from build123d import *

# Parameters (mm, degrees)
SKETCH1_W                 = 270.7
SKETCH1_H                 = 127
SKETCH1_R                 = 1.6
WALL_DEPTH                = 6.35
SKETCH5_R                 = 3.96875
RODSUPPORTCUTOUT_DEPTH    = 3.175
SUPPORTPATTERN_COUNT      = 7
SUPPORTPATTERN_PITCH      = 36.65
SUPPORTPATTERN_COUNT_DIR2 = 5
SUPPORTPATTERN_PITCH_DIR2 = 19.05


with BuildPart() as part:
    # Sketch1 → Wall (new body)
    with BuildSketch(Plane.XY):
        with Locations((135.35, 63.5)):
            Rectangle(SKETCH1_W, SKETCH1_H)
        with Locations((12.35, 105)):
            Circle(SKETCH1_R, mode=Mode.SUBTRACT)
        with Locations(Location((258.35, 105, 0), (0, 0, 180))):
            Circle(SKETCH1_R, mode=Mode.SUBTRACT)
        with Locations((258.35, 22)):
            Circle(SKETCH1_R, mode=Mode.SUBTRACT)
        with Locations(Location((12.35, 22, 0), (0, 0, 180))):
            Circle(SKETCH1_R, mode=Mode.SUBTRACT)
    extrude(amount=WALL_DEPTH)

    # Sketch5 → RodSupportCutout (cut)
    with BuildSketch(Plane.XY.offset(6.35)):
        with Locations(Location((25.4, 101.6, 0), (0, 0, 180))):
            Circle(SKETCH5_R)
    rodsupportcutout = extrude(amount=-RODSUPPORTCUTOUT_DEPTH, mode=Mode.SUBTRACT)

    # SupportPattern: RodSupportCutout 7 × 5
    with Locations(*[(i * SUPPORTPATTERN_PITCH, -j * SUPPORTPATTERN_PITCH_DIR2, 0) for i in range(SUPPORTPATTERN_COUNT) for j in range(SUPPORTPATTERN_COUNT_DIR2) if (i, j) != (0, 0)]):
        add(rodsupportcutout, mode=Mode.SUBTRACT)


solid = part.part
Read the model definition and answer for the solid it produces. Units are mm, in the model's axes. A direction names the side the tool comes from. Round coordinates to 2 decimals unless told otherwise and drop trailing zeros. Order: outer loops, then holes, each group sorted by start corner. A loop starts at its lowest first (then second) coordinate and runs counter-clockwise, first axis right, second up. Notation, with made-up numbers: (69, 32.25) - (93, 32.25) arc R19 ccw to (93, 55.25) - close; hole circle Ø7 at (40, -23). An arc over 180 degrees is marked (long way). Use one line per item in the form item = value. Start each with the question number.
(1) Determine the mould class of faces 3 (the face through (133, 0, 3)), 4 (the face through (101.625, 60.818, 4.785)), 5 (the face through (270.7, 63, 3)) for opening direction X: +X half, -X half, draft (parallel to the pull), parting line (faces both ways), or undercut.
(2) The part is cut by section C-C (x = 209.5). Give the vertices of the cut face in (y, z) (3 decimals), then the cut area to 3 significant figures.
(3) The part is cut by section A-A (x = 98.7). Give the vertices of the cut face in (y, z) (3 decimals).
(4) For faces 1 (the face through (133, 127, 3)), 2 (the face through (209, 44, 3.175)), determine the directions among +Z, -Z, +X, -X, +Y, -Y from which every point of the face is accessible in a straight line to the end or side of a thin tool.
(5) Flat-ended cylindrical pins translate along their axes: pin 1 Ø6.5 at (x, y) = (246, 103) entering from +Z; pin 2 Ø6.5 at (x, y) = (172, 25.4) entering from +Z (3 decimals). Find the tip coordinate at first contact, or state that the pin passes through.
(6) Find the intervals of material crossed by line 1 along Y through (x, z) = (136, 5.25); line 2 along Y through (x, z) = (208.65, 4.85); line 3 along X through (y, z) = (105, 2), in increasing order. Write a range as from..to.
Checked values:
q1.face_3 = draft
q1.face_4 = undercut
q1.face_5 = +X half
q2.outline = (0, 0) - (127, 0) - (127, 6.35) - (105.477, 6.35) - (105.477, 3.175) - (97.723, 3.175) - (97.723, 6.35) - (86.427, 6.35) - (86.427, 3.175) - (78.673, 3.175) - (78.673, 6.35) - (67.377, 6.35) - (67.377, 3.175) - (59.623, 3.175) - (59.623, 6.35) - (48.327, 6.35) - (48.327, 3.175) - (40.573, 3.175) - (40.573, 6.35) - (29.277, 6.35) - (29.277, 3.175) - (21.523, 3.175) - (21.523, 6.35) - (0, 6.35) - close
q2.area = 683 mm^2
q3.outline = (0, 0) - (127, 0) - (127, 6.35) - (105.569, 6.35) - (105.569, 3.175) - (97.631, 3.175) - (97.631, 6.35) - (86.519, 6.35) - (86.519, 3.175) - (78.581, 3.175) - (78.581, 6.35) - (67.469, 6.35) - (67.469, 3.175) - (59.531, 3.175) - (59.531, 6.35) - (48.419, 6.35) - (48.419, 3.175) - (40.481, 3.175) - (40.481, 6.35) - (29.369, 6.35) - (29.369, 3.175) - (21.431, 3.175) - (21.431, 6.35) - (0, 6.35) - close
q4.face_1 = +Z, -Z, +X, -X, +Y
q4.face_2 = +Z
q5.pin_1 = 6.35
q5.pin_2 = 3.175
q6.line_1 = 0..21.48, 29.32..40.53, 48.37..59.58, 67.42..78.63, 86.47..97.68, 105.52..127
q6.line_2 = 0..21.43, 29.37..40.48, 48.42..59.53, 67.47..78.58, 86.52..97.63, 105.57..127
q6.line_3 = 0..10.75, 13.95..256.75, 259.95..270.7
